Geometry: see drawing. Coordinates: mm, zero at the bounding-box minimum. A direction names the side the tool comes from. Coordinates: 2 decimals unless noted, no trailing zeros. Loops run counter-clockwise (first coordinate to the right, second up) from the corner with the lowest first, then second, coordinate; pieces in that order, holes last. Notation, with made-up numbers: (75.25, 64.25) -> (112.25, 64.25) arc R15 cw to (112.25, 68.25) -> close; hole circle Ø7 at (-24.75, -25). An arc over 180 degrees is marked (long way). One line per item, written item: value. Start each with the question number.
Item 1: Section query D-D on z = 8.5. Return loops of the section in (x, y), then the cut area to 3 significant figures.
Item 2: Contact query for flat-ended pins moving along their axis: pin 1 Ø4.5 at (x, y) = (10.5, 11) entering from -Z; pin 2 Ø8 at (x, z) = (41, 2.5) entering from +Y; pin 3 Ø8 at (x, y) = (17, 20.5) entering from +Z. Output: stop coordinate, or through.
Item 3: Section query B-B on z = 12.7. Return loops of the section in (x, y).
Item 4: Section query C-C on x = 12.5. Return loops of the section in (y, z).
Item 5: Set-up query: the marked faces 1, 2 and 3. Return all of +Z, -Z, +X, -X, +Y, -Y with unobstructed straight access to the full face (end or side cutting, diameter ignored); none if empty.
Item 6: Ray query, probe 1 along X at (y, z) = (11.5, 3.75); probe 2 along Z at (x, y) = (23, 9.5); probe 3 along Z at (x, y) = (17, 3.75). Return the intervals inside material, ascending. Write a range as from..to.
Item 7: Section query A-A on y = 12.7. Return loops of the section in (x, z), then the cut area to 3 significant figures.
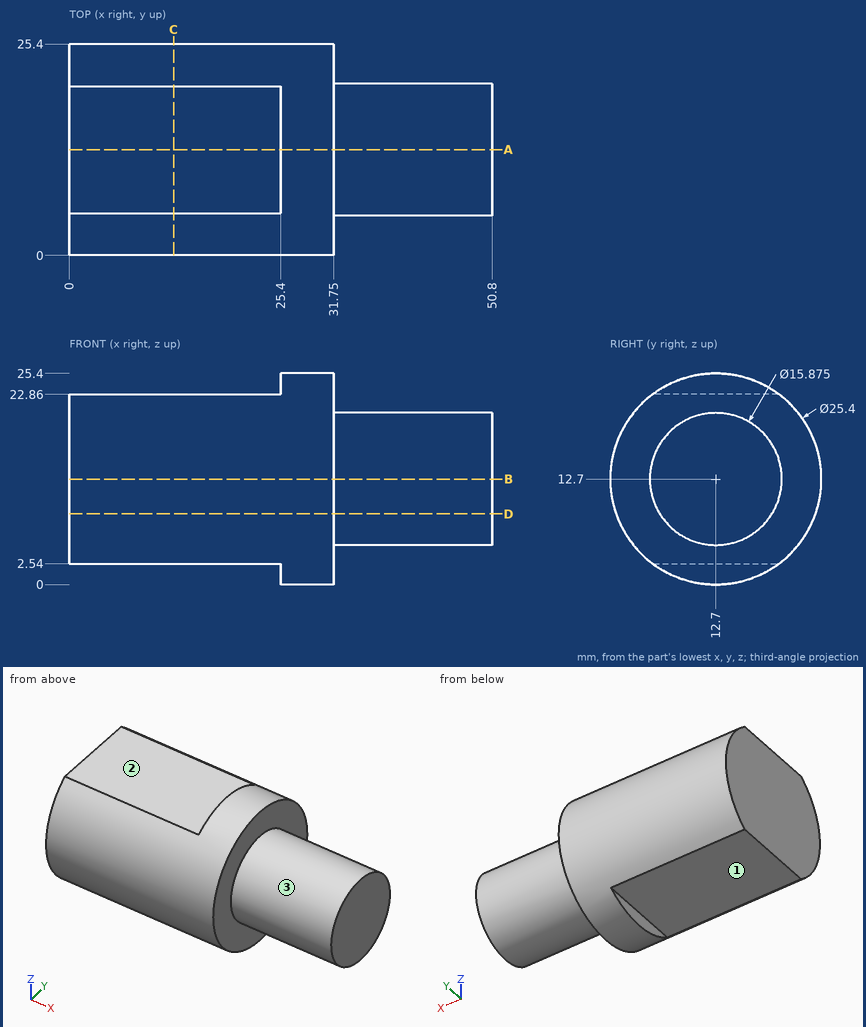
Reply:
1. outline: (0, 0.71) -> (31.75, 0.71) -> (31.75, 5.96) -> (50.8, 5.96) -> (50.8, 19.44) -> (31.75, 19.44) -> (31.75, 24.69) -> (0, 24.69) -> close
1. area: 1,020 mm²
2. pin 1: stops at z = 2.54
2. pin 2: stops at y = 17.66
2. pin 3: stops at z = 22.86
3. outline: (0, 0) -> (31.75, 0) -> (31.75, 4.76) -> (50.8, 4.76) -> (50.8, 20.64) -> (31.75, 20.64) -> (31.75, 25.4) -> (0, 25.4) -> close
4. outline: (5.08, 2.54) -> (20.32, 2.54) arc R12.7 ccw to (20.32, 22.86) -> (5.08, 22.86) arc R12.7 ccw to start
5. face 1: -Z, -X, +Y, -Y
5. face 2: +Z, -X, +Y, -Y
5. face 3: +X
6. probe 1: x = 0..31.75
6. probe 2: z = 2.54..22.86
6. probe 3: z = 3.69..21.71
7. outline: (0, 2.54) -> (25.4, 2.54) -> (25.4, 0) -> (31.75, 0) -> (31.75, 4.76) -> (50.8, 4.76) -> (50.8, 20.64) -> (31.75, 20.64) -> (31.75, 25.4) -> (25.4, 25.4) -> (25.4, 22.86) -> (0, 22.86) -> close
7. area: 980 mm²
